Can you work these out from the drawing? Everything is in mm from the part's minimum corner. Round coordinates to 2 decimals unless told otherwise and drop trailing zeros. Loops run counter-clockwise (first coordinate to the right, second up) from the corner with the lowest first, then second, coordinate; pieces in that order, holes last. Notation, with made-up numbers: M 41.5,9 L 58.5,9 A13 cw 58.5,19 Z; hole C -6,85.25 d11. An arc over 180 degrees is marked long. Use a Markdown table: item, result.
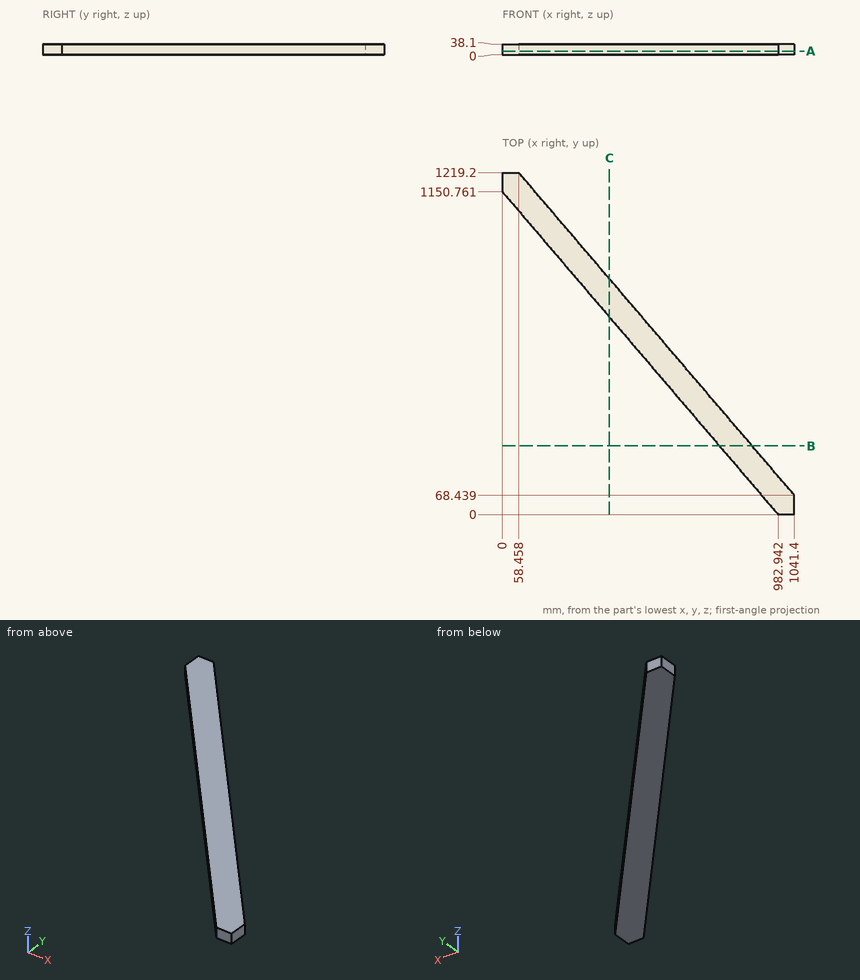
Q1. I need wall thicknesses on line 1 (X direction, y = 250, z = 30.5); line 2 (X direction, y = 451, z = 13.5); line 3 (Y direction, x = 427.5, z = 9.5). Which ranges of each line are inside material? Lowest first, please. Write a range as from..to.
Return value:
| item | result |
|---|---|
| line 1 | x = 769.4..886.32 |
| line 2 | x = 597.71..714.63 |
| line 3 | y = 650.27..787.15 |
Q2. Will these pins go through, and if not, where does the flat tip stop? P1, Ø6, axis at y = 999.5, z = 30, coming from the -X side; P2, Ø10, axis at x = 645, z = 5.5, coming from the +Y side; P3, Ø6, axis at y = 870.5, z = 20.5, coming from the +X side.
Return value:
| item | result |
|---|---|
| P1 | stops at x = 126.64 |
| P2 | stops at y = 538.37 |
| P3 | stops at x = 358.87 |
Q3. Imagine slicing it at C-C, the plane x = 381. Please give me the cut outline in (y, z), then the cut area to 4 significant figures.
Return value:
| item | result |
|---|---|
| outline | M 704.71,0 L 841.59,0 L 841.59,38.1 L 704.71,38.1 Z |
| area | 5,215 mm^2 |
Q4. Imagine slicing it at A-A, the plane z = 13. Please give me the cut outline in (x, y), then the cut area to 3 significant figures.
Return value:
| item | result |
|---|---|
| outline | M 0,1150.76 L 982.94,0 L 1041.4,0 L 1041.4,68.44 L 58.46,1219.2 L 0,1219.2 Z |
| area | 139,000 mm^2 |
Q5. Imagine slicing it at B-B, the plane y = 245. Please give me the cut outline in (x, z), then the cut area to 3 significant figures.
Return value:
| item | result |
|---|---|
| outline | M 773.67,0 L 890.59,0 L 890.59,38.1 L 773.67,38.1 Z |
| area | 4,450 mm^2 |
